```python
from build123d import *

# Parameters (mm, degrees)
SKETCH1_W           = 88
SKETCH1_H           = 88
BOSS_EXTRUDE1_DEPTH = 4
FILLET1_R           = 10
SKETCH2_R           = 2.15
CUT_EXTRUDE1_DEPTH  = 5
SKETCH3_W           = 200
SKETCH3_H           = 41
BOSS_EXTRUDE2_DEPTH = 4
SKETCH5_R           = 2.5
CUT_EXTRUDE2_DEPTH  = 5


with BuildPart() as part:
    # Sketch1 → Boss-Extrude1 (new body)
    with BuildSketch(Plane(origin=(0, 0, 0), x_dir=(1, 0, 0), z_dir=(0, 1, 0))):
        Rectangle(SKETCH1_W, SKETCH1_H)
    extrude(amount=BOSS_EXTRUDE1_DEPTH)

    # Fillet1
    fillet1_edges = [part.edges().sort_by_distance(p)[0] for p in [
        (-44, 2, -44),
        (44, 2, -44),
        (44, 2, 44),
        (-44, 2, 44),
    ]]
    fillet(fillet1_edges, radius=FILLET1_R)

    # Sketch2 → Cut-Extrude1 (cut, through all)
    with BuildSketch(Plane(origin=(0, 4, 0), x_dir=(1, 0, 0), z_dir=(0, 1, 0))):
        with Locations((34, 34)):
            Circle(SKETCH2_R)
        with Locations((-34, 34)):
            Circle(SKETCH2_R)
        with Locations((34, -34)):
            Circle(SKETCH2_R)
        with Locations((-34, -34)):
            Circle(SKETCH2_R)
    extrude(amount=-CUT_EXTRUDE1_DEPTH, mode=Mode.SUBTRACT)

    # Sketch3 → Boss-Extrude2 (add)
    with BuildSketch(Plane(origin=(0, 0, 0), x_dir=(1, 0, 0), z_dir=(0, 1, 0))):
        Rectangle(SKETCH3_W, SKETCH3_H)
    extrude(amount=BOSS_EXTRUDE2_DEPTH)

    # Sketch5 → Cut-Extrude2 (cut, through all)
    with BuildSketch(Plane.XZ):
        with Locations((-66, 13)):
            Circle(SKETCH5_R)
        with Locations((-66, -13)):
            Circle(SKETCH5_R)
        with Locations((-94, -13)):
            Circle(SKETCH5_R)
        with Locations((-94, 13)):
            Circle(SKETCH5_R)
    cut_extrude2 = extrude(amount=-CUT_EXTRUDE2_DEPTH, mode=Mode.SUBTRACT)

    # Mirror1: Cut-Extrude2 across plane
    add(cut_extrude2.mirror(Plane(origin=(0, 0, 0), x_dir=(0, 0, 1), z_dir=(1, 0, 0))), mode=Mode.SUBTRACT)


solid = part.part
```
Build history of the part. All positions in model axes, mm. A direction names the side the tool comes from. Round coordinates to 2 decimals unless told otherwise and drop trailing zeros. Write each loop counter-clockwise with the first axis right and the second up, starting at its lowest first coordinate (ties: lowest second). Pieces come first, ordered by that corner, then holes. Notation, with made-up numbers: (-10, -11) -> (31, -11) arc R16 cw to (31, 8) -> close; hole circle Ø9 at (46.25, -37). An arc over 180 degrees is marked (long way). Put each result on its own line as item: value.
Item 1: Slice it at B-B, the plane x = -94. Give the cut face in (y, z), plus the area to 3 significant figures.
Here are the results:
outline: (0, -20.5) -> (4, -20.5) -> (4, -15.5) -> (0, -15.5) -> close; (0, -10.5) -> (4, -10.5) -> (4, 10.5) -> (0, 10.5) -> close; (0, 15.5) -> (4, 15.5) -> (4, 20.5) -> (0, 20.5) -> close
area: 124 mm^2
Item 2: Two-plate mould, pull along X, no slides. Class faces 4 (the face through (41.15, 2.03, -40.99)), 5 (the face through (-32.84, 2.03, 32.19)), 6 (the face through (0, 2, -44)): pulls with the +X half, pulls with the -X half, needs draft (parallel to the pull), parting line crosses it, or undercut.
Here are the results:
face 4: pulls with the +X half
face 5: undercut
face 6: needs draft
Item 3: Slice it at C-C, the plane x = -49. Give the cut face in (y, z).
Here are the results:
outline: (0, -20.5) -> (4, -20.5) -> (4, 20.5) -> (0, 20.5) -> close
Item 4: Flat gauge pin, fed straight in: P1, Ø1.2, axis at y = 1.5, z = 27, coming from the -X side. Where does the tip first touch, or does it go through?
Here are the results:
P1: stops at x = -44
Item 5: Slice it at A-A, the plane z = -13. Give the cut face in (x, y), plus the area to 3 significant figures.
Here are the results:
outline: (-100, 0) -> (-96.5, 0) -> (-96.5, 4) -> (-100, 4) -> close; (-91.5, 0) -> (-68.5, 0) -> (-68.5, 4) -> (-91.5, 4) -> close; (-63.5, 0) -> (63.5, 0) -> (63.5, 4) -> (-63.5, 4) -> close; (68.5, 0) -> (91.5, 0) -> (91.5, 4) -> (68.5, 4) -> close; (96.5, 0) -> (100, 0) -> (100, 4) -> (96.5, 4) -> close
area: 720 mm^2
Item 6: Wall check: probe 1 along Z at (x, y) = (66, 1.45); probe 2 along X at (y, z) = (1.25, -34); probe 3 along X at (y, z) = (3.5, -29.5). Give the ranges that are in metal, low to high. Write a range as from..to.
Here are the results:
probe 1: z = -20.5..-15.5, -10.5..10.5, 15.5..20.5
probe 2: x = -44..-36.15, -31.85..31.85, 36.15..44
probe 3: x = -44..44
Item 7: Slice it at D-D, the plane z = 27. Give the cut face in (x, y), plus the area to 3 significant figures.
Here are the results:
outline: (-44, 0) -> (44, 0) -> (44, 4) -> (-44, 4) -> close
area: 352 mm^2
Item 8: Tool access for faces 1 (the face through (-96, 2, -14.5)), 2 (the face through (-72, 2, 20.5)), 3 (the face through (-44, 2, -27)): list every direction of +Z, -Z, +X, -X, +Y, -Y with a clear straight run to the whole face (end or side of a thin tool).
Here are the results:
face 1: +Y, -Y
face 2: +Z, -X, +Y, -Y
face 3: -Z, -X, +Y, -Y
